from build123d import *

# Parameters (mm, degrees)
F0_R      = 6
F1_DEPTH  = 25
F2_R      = 7
F3_DEPTH  = 2
F3_FACE_R = 7
F5_R      = 3.5
F7_DEPTH  = 7


with BuildPart() as f1:
    # F0 (on Top) → F1 (new body)
    with BuildSketch(Plane.XY):
        Circle(F0_R)
    extrude(amount=F1_DEPTH)

    # F2 (on face) → F3 (join)
    with BuildSketch(Plane.XY.offset(25)):
        Circle(F2_R)
    extrude(amount=F3_DEPTH)

    # F3_face (on face) → F6 section 0
    with BuildSketch(Plane.XY.offset(27)):
        Circle(F3_FACE_R)
    # F5 (on offset) → F6 section 1
    with BuildSketch(Plane.XY.offset(47)):
        Circle(F5_R)
    loft()

    # F7 (add): a face of the model
    f7_faces = [f1.faces().sort_by_distance(p)[0] for p in [
        (0, 0, 47),
    ]]
    extrude(f7_faces, amount=F7_DEPTH)

    # F8 (on face) → F9 (revolve)
    with BuildSketch(Plane.XY.offset(54)):
        with BuildLine():
            Line((0.407853673, -3.4761552585), (0, 0))
            Line((0, 0), (-0.407853673, 3.4761552585))
            ThreePointArc((-0.407853673, 3.4761552585), (-3.4761552585, -0.407853673), (0.407853673, -3.4761552585))
        make_face()
    revolve(axis=Axis((0.2039268365, -1.7380776293, 54), (0.1165296209, -0.9931872167, 0)))


solid = f1.part
Input: part model. Units: mm. Frame: model coordinates. A direction names the side the tool comes from. Coordinates: 2 decimals unless noted, no trailing zeros. Order: outer loops, then holes, each group sorted by start corner. A loop starts at its lowest first (then second) coordinate and runs counter-clockwise, first axis right, second up. Notation, with made-up numbers: M -9.5,-9.5 L 17.5,-9.5 A37 ccw 17.5,28.5 Z; hole C 61,-26.75 d2. An arc over 180 degrees is marked long. Answer as CSV lines item,"result".
1. First-contact query: P1, Ø1.5, axis at x = -4.5, z = 20.5, coming from the +Y side; P2, Ø1.5, axis at y = 4, z = 31.5, coming from the +X side; P3, Ø6, axis at y = -4, z = 26.5, coming from the +X side. Flat tips, straight axial feed; report the tip coordinate or a pass-through.
Reported:
P1,"y = 4.68"
P2,"x = 5.32"
P3,"x = 6.93"
2. Section B-B (z = 31). Return the cut outline in (x, y).
Reported:
outline,"C 0,0 d12.6"
3. Material intervals for line 1 (X direction, y = 1.5, z = 19.5); line 2 (X direction, y = 2, z = 3); line 3 (Y direction, x = 1, z = 10), sorted ascending. Write a range as from..to.
Reported:
line 1,"-5.81..5.81"
line 2,"-5.66..5.66"
line 3,"-5.92..5.92"
4. Access query for faces 1 (the cylindrical face through (3.233, -1.341, 50.451)), 2 (the cylindrical face through (-6, 0, 12)), 3 (the cylindrical face through (6.466, -2.681, 25.986)). Directions: +Z, -Z, +X, -X, +Y, -Y. A direction counts if a zero-diameter tool reaches every point of the face in a straight line with its end or side. Return the directions, or none.
Reported:
face 1,"+Z"
face 2,"-Z"
face 3,"+Z, -Z"
5. Section A-A (z = 50). Return the cut outline in (x, y).
Reported:
outline,"C 0,0 d7"
